Read the model definition and answer for the solid it produces. Units are mm, in the model's axes. Face numbers are marked on the shaded views. A direction names the side the tool comes from. Coordinates: 2 decimals unless noted, no trailing zeros. Write each loop counter-clockwise with the first axis right and the second up, starting at its lowest first coordinate (ties: lowest second). Pieces come first, ordered by that corner, then holes. Notation, with made-up numbers: (35.5, -1.75) -> (94.5, -1.75) arc R18 ccw to (94.5, 10.25) -> close; hole circle Ø1 at (-27, 28.5). An arc over 180 degrees is marked (long way). Answer in a Markdown table with one row per item. Add a question column.
Item 1: Section D-D on z = 10.5 is taken. Write down the section's boundary in (x, y), then the cut area to 3 significant figures.
Item 2: Section A-A on y = 0 is taken. Write down the section's boundary in (x, z).
Item 3: Which of the six approach directions +Z, -Z, +X, -X, +Y, -Y give full straight-line access (tool end or side, diameter ignored) to the marked faces 1, 2, 3, 4 and 5?
Item 4: For a pull along Z with two mould halves and no side action, classify the marked faces 6, 7, 8 and 9 as +Z half, -Z half, draft (parallel to the pull), parting line (faces both ways), or undercut.
Item 5: Section C-C on z = -7 is taken. Write down the section's boundary in (x, y), then the cut area to 3 significant figures.
Item 6: Given pin 1 Ø8 at (y, z) = (33, 17) entering from -X; pin 2 Ø2 at (x, y) = (-14.5, -0.5) entering from -Z; pin 3 Ø6 at (y, z) = (33, 15.5) entering from +X, each flat-ended and moving along its own axis, determine where each tip first touches the part or whether it passes through.
Item 7: Section B-B on x = 6 is taken. Write down the section's boundary in (y, z).
Item 8: Straight lines are drawn through the part: line 1 (Y direction, x = 0, z = 18); line 2 (Y direction, x = 0, z = 4.5); line 3 (Z direction, x = -14, y = -5). For each, find the intervals that lie inside material, in ascending order. Write a range as from..to.
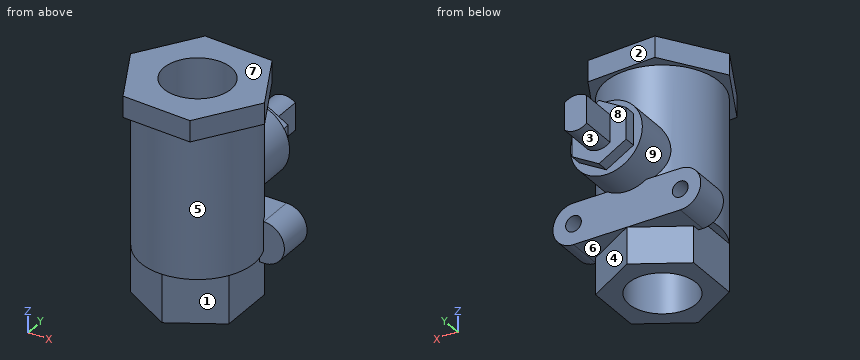
```python
from build123d import *

# Parameters (mm, degrees)
SKETCH1_R                = 15.0114
BOSS_EXTRUDE1_DEPTH      = 38.1
BOSS_EXTRUDE2_DEPTH      = 5.588
BOSS_EXTRUDE3_DEPTH      = 12.7
BOSS_EXTRUDE4_DEPTH      = 9.5504
SKETCH4_R                = 8.89
CUT_EXTRUDE1_DEPTH       = 62.91098247
BOSS_EXTRUDE5_DEPTH      = 8.636
BOSS_EXTRUDE5_DEPTH_BACK = 5.08
SKETCH6_R                = 9.525
BOSS_EXTRUDE6_DEPTH      = 3.1115
SKETCH8_W                = 5.842
SKETCH8_H                = 7.231465202
BOSS_EXTRUDE7_DEPTH      = 9.8298
SKETCH9_R                = 2.08915
CUT_EXTRUDE2_DEPTH       = 8.89


with BuildPart() as part:
    # Sketch1 → Boss-Extrude1 (new body)
    with BuildSketch(Plane.XY):
        with Locations(Location((0, 0, 0), (0, 0, 180))):
            Circle(SKETCH1_R)
    extrude(amount=BOSS_EXTRUDE1_DEPTH)

    # Sketch2 → Boss-Extrude2 (add)
    with BuildSketch(Plane.XY.offset(38.1)):
        Polygon((-8.314485622, 16.42722286), (-18.383635121, 1.013055662), (-10.069149499, -15.414167198), (8.314485622, -16.42722286), (18.383635121, -1.013055662), (10.069149499, 15.414167198), align=None)
    extrude(amount=BOSS_EXTRUDE2_DEPTH)

    # Sketch3 → Boss-Extrude3 (add)
    with BuildSketch(Plane(origin=(0, 0, 0), x_dir=(-1, 0, 0), z_dir=(0, 0, -1))):
        Polygon((0, 15.0114), (-13.000253746, 7.5057), (-13.000253746, -7.5057), (0, -15.0114), (13.000253746, -7.5057), (13.000253746, 7.5057), align=None)
    extrude(amount=BOSS_EXTRUDE3_DEPTH)

    # Sketch5 → Boss-Extrude4 (add)
    with BuildSketch(Plane(origin=(0, 15.0114, 0), x_dir=(1, 0, 0), z_dir=(0, 1, 0))):
        with BuildLine():
            Line((-14.1351, 3.048), (14.1351, 3.048))
            ThreePointArc((14.1351, 3.048), (19.5834, -2.4003), (14.1351, -7.8486))
            Line((14.1351, -7.8486), (-14.1351, -7.8486))
            ThreePointArc((-14.1351, -7.8486), (-19.5834, -2.4003), (-14.1351, 3.048))
        make_face()
    extrude(amount=-BOSS_EXTRUDE4_DEPTH)

    # Sketch4 → Cut-Extrude1 (cut, through all)
    with BuildSketch(Plane(origin=(0, 0, -12.7), x_dir=(-1, 0, 0), z_dir=(0, 0, -1))):
        Circle(SKETCH4_R)
    extrude(amount=-CUT_EXTRUDE1_DEPTH, mode=Mode.SUBTRACT)

    # Sketch6 → Boss-Extrude5 (add, two sides: drawn at the far end of the back side and taken through both)
    with BuildSketch(Plane(origin=(0, 15.0114, 0), x_dir=(1, 0, 0), z_dir=(0, 1, 0)).offset(-BOSS_EXTRUDE5_DEPTH_BACK)):
        with Locations(Location((0, -15.875, 0), (0, 0, 180))):
            Circle(SKETCH6_R)
    extrude(amount=BOSS_EXTRUDE5_DEPTH + BOSS_EXTRUDE5_DEPTH_BACK)

    # Sketch7 → Boss-Extrude6 (add)
    with BuildSketch(Plane(origin=(0, 23.6474, 0), x_dir=(1, 0, 0), z_dir=(0, 1, 0))):
        Polygon((0, -7.57478159), (-7.1882, -11.724890795), (-7.1882, -20.025109205), (0, -24.17521841), (7.1882, -20.025109205), (7.1882, -11.724890795), align=None)
    extrude(amount=BOSS_EXTRUDE6_DEPTH)

    # Sketch8 → Boss-Extrude7 (add)
    with BuildSketch(Plane(origin=(0, 26.7589, 0), x_dir=(1, 0, 0), z_dir=(0, 1, 0))):
        with Locations((0, -15.875)):
            Rectangle(SKETCH8_W, SKETCH8_H)
        with BuildLine():
            ThreePointArc((2.921, -12.259267399), (0, -11.2268), (-2.921, -12.259267399))
            Line((-2.921, -12.259267399), (2.921, -12.259267399))
        make_face()
        with BuildLine():
            Line((2.921, -19.490732601), (-2.921, -19.490732601))
            ThreePointArc((-2.921, -19.490732601), (0, -20.5232), (2.921, -19.490732601))
        make_face()
    extrude(amount=BOSS_EXTRUDE7_DEPTH)

    # Sketch9 → Cut-Extrude2 (cut)
    with BuildSketch(Plane(origin=(0, 15.0114, 0), x_dir=(1, 0, 0), z_dir=(0, 1, 0))):
        with Locations(Location((14.1351, -2.4003, 0), (0, 0, 180))):
            Circle(SKETCH9_R)
        with Locations(Location((-14.1351, -2.4003, 0), (0, 0, 180))):
            Circle(SKETCH9_R)
    extrude(amount=-CUT_EXTRUDE2_DEPTH, mode=Mode.SUBTRACT)


solid = part.part
```
Results below:
| question | item | result |
|---|---|---|
| 1 | outline | (-7.86, 12.79) arc R15.01 ccw (long way) to (7.86, 12.79) -> (7.86, 23.65) -> (5.07, 23.65) -> (5.07, 26.76) -> (-5.07, 26.76) -> (-5.07, 23.65) -> (-7.86, 23.65) -> close; hole circle Ø17.78 at (0, 0) |
| 1 | area | 638 mm2 |
| 2 | outline | (-17.87, 38.1) -> (-15.01, 38.1) -> (-15.01, 0) -> (-13, 0) -> (-13, -12.7) -> (-8.89, -12.7) -> (-8.89, 43.69) -> (-17.87, 43.69) -> close; (8.89, -12.7) -> (13, -12.7) -> (13, 0) -> (15.01, 0) -> (15.01, 38.1) -> (17.87, 38.1) -> (17.87, 43.69) -> (8.89, 43.69) -> close |
| 3 | face 1 | -Z, +X, -Y |
| 3 | face 2 | +Z, +X, +Y |
| 3 | face 3 | -Z, +Y |
| 3 | face 4 | -Z, +X, +Y |
| 3 | face 5 | none |
| 4 | face 6 | -Z half |
| 4 | face 7 | +Z half |
| 4 | face 8 | draft |
| 4 | face 9 | undercut |
| 5 | outline | (-13, -7.51) -> (0, -15.01) -> (13, -7.51) -> (13, 7.51) -> (0, 15.01) -> (-13, 7.51) -> close; hole circle Ø17.78 at (0, 0) |
| 5 | area | 337 mm2 |
| 6 | pin 1 | stops at x = -2.92 |
| 6 | pin 2 | stops at z = 0 |
| 6 | pin 3 | stops at x = 2.92 |
| 7 | outline | (-16.3, 38.1) -> (-13.76, 38.1) -> (-13.76, 0) -> (-11.55, 0) -> (-11.55, -12.7) -> (-6.56, -12.7) -> (-6.56, 43.69) -> (-16.3, 43.69) -> close; (6.56, -12.7) -> (11.55, -12.7) -> (11.55, -3.05) -> (15.01, -3.05) -> (15.01, 7.85) -> (13.76, 7.85) -> (13.76, 8.48) -> (23.65, 8.48) -> (23.65, 11.04) -> (26.76, 11.04) -> (26.76, 20.71) -> (23.65, 20.71) -> (23.65, 23.27) -> (13.76, 23.27) -> (13.76, 38.1) -> (15.64, 38.1) -> (15.64, 43.69) -> (6.56, 43.69) -> close |
| 8 | line 1 | y = -15.01..-8.89, 8.89..36.59 |
| 8 | line 2 | y = -15.01..-8.89, 8.89..15.01 |
| 8 | line 3 | z = 0..43.69 |
